CAD build for the part. Positions are in the model's coordinates, mm. A direction names the side the tool comes from. Coordinates: 2 decimals unless noted, no trailing zeros. Write each loop counter-clockwise with the first axis right and the second up, starting at its lowest first coordinate (ties: lowest second). Pieces come first, ordered by that corner, then holes. Notation, with made-up numbers: (18.25, 38) - (56.25, 38) arc R4 cw to (56.25, 44) - close; hole circle Ø6 at (17.5, -9). An arc over 180 degrees is marked (long way). Answer in a Markdown table with one row per item. Add a question column.
Q1. Band-saw the part on B-B (y = 9). List the corners of the cut face in (x, z), and give its area (3 significant figures).
Q2. Band-saw the part on C-C (z = 0). List the corners of the cut face in (x, y).
Q3. Drill centre lines: line 1 along X through (y, z) = (5.75, 0); line 2 along X through (y, z) = (2.75, 5.75); line 3 along Y through (x, z) = (16, 7). Where is each one in solid material? Low to high. Write a range as from..to.
Q4. Band-saw the part on A-A (x = 10). List the corners of the cut face in (y, z).
Q5. Two-plate mould, pull along Z, no slides. Class faces 5 (the cylindrical face through (4.5, 3, -7.5)), 6 (the flat face through (0, 1, 10)), 7 (the flat face through (-20, 1, 0)): +Z half, -Z half, draft (parallel to the pull), parting line (faces both ways), or undercut.
Q6. Pin check, flat tips, straight feed: pin 1 (6 mm diameter, centred on x = -11, y = 12, fed in from -Z); pin 2 (3.5 mm diameter, centred on x = 0, z = -8, fed in from +Y); pin 3 (4 mm diameter, centred on x = -11, z = -3.5, fed in from +Y). Stop position of each tip, or through.
Q7. 3-axis set-ups, long thin cutter, end or side, ignore diameter. For faces 1 (the cylindrical face through (-17.32, 7.92, -1.63)), 2 (the flat face through (0, 3, -9)), 3 (the flat face through (0, 4, -8)), 4 (the flat face through (20, 1, 0)): which of +Z, -Z, +X, -X, +Y, -Y reach the whole face in a straight line?
```python
from build123d import *

# Parameters (mm, degrees)
SKETCH1_W           = 40
SKETCH1_H           = 20
BOSS_EXTRUDE1_DEPTH = 2
SKETCH2_R           = 7.5
BOSS_EXTRUDE2_DEPTH = 12
SKETCH3_R           = 6.5
CUT_EXTRUDE1_DEPTH  = 12
SKETCH7_R           = 6.5
CUT_EXTRUDE2_DEPTH  = 12
BOSS_EXTRUDE3_DEPTH = 2


with BuildPart() as part:
    # Sketch1 → Boss-Extrude1 (new body)
    with BuildSketch(Plane(origin=(0, 0, 0), x_dir=(1, 0, 0), z_dir=(0, 1, 0))):
        Rectangle(SKETCH1_W, SKETCH1_H)
    extrude(amount=BOSS_EXTRUDE1_DEPTH)

    # Sketch2 → Boss-Extrude2 (add)
    with BuildSketch(Plane(origin=(0, 2, 0), x_dir=(1, 0, 0), z_dir=(0, 1, 0))):
        with Locations(Location((-10, 0, 0), (0, 0, 270))):
            Circle(SKETCH2_R)
        with Locations(Location((10, 0, 0), (0, 0, 270))):
            Circle(SKETCH2_R)
    extrude(amount=BOSS_EXTRUDE2_DEPTH)

    # Sketch3 → Cut-Extrude1 (cut)
    with BuildSketch(Plane(origin=(0, 14, 0), x_dir=(1, 0, 0), z_dir=(0, 1, 0))):
        with Locations(Location((-10, 0, 0), (0, 0, 270))):
            Circle(SKETCH3_R)
    extrude(amount=-CUT_EXTRUDE1_DEPTH, mode=Mode.SUBTRACT)

    # Sketch7 → Cut-Extrude2 (cut)
    with BuildSketch(Plane(origin=(0, 14, 0), x_dir=(1, 0, 0), z_dir=(0, 1, 0))):
        with Locations(Location((10, 0, 0), (0, 0, 270))):
            Circle(SKETCH7_R)
    extrude(amount=-CUT_EXTRUDE2_DEPTH, mode=Mode.SUBTRACT)

    # Sketch9 → Boss-Extrude3 (add)
    with BuildSketch(Plane(origin=(0, 2, 0), x_dir=(1, 0, 0), z_dir=(0, 1, 0))):
        with BuildLine():
            Line((-3, 9), (3, 9))
            ThreePointArc((3, 9), (4.5, 7.5), (3, 6))
            Line((3, 6), (-3, 6))
            ThreePointArc((-3, 6), (-4.5, 7.5), (-3, 9))
        make_face()
    extrude(amount=BOSS_EXTRUDE3_DEPTH)


solid = part.part
```
Checked values:
| question | item | result |
|---|---|---|
| 1 | outline | circle Ø15 at (-10, 0); circle Ø15 at (10, 0); hole circle Ø13 at (-10, 0); hole circle Ø13 at (10, 0) |
| 1 | area | 88.0 mm² |
| 2 | outline | (-20, 0) - (20, 0) - (20, 2) - (17.5, 2) - (17.5, 14) - (16.5, 14) - (16.5, 2) - (3.5, 2) - (3.5, 14) - (2.5, 14) - (2.5, 2) - (-2.5, 2) - (-2.5, 14) - (-3.5, 14) - (-3.5, 2) - (-16.5, 2) - (-16.5, 14) - (-17.5, 14) - (-17.5, 2) - (-20, 2) - close |
| 3 | line 1 | x = -17.5..-16.5, -3.5..-2.5, 2.5..3.5, 16.5..17.5 |
| 3 | line 2 | x = -14.82..-13.03, -6.97..-5.18, 5.18..6.97, 13.03..14.82 |
| 3 | line 3 | y = 0..2 |
| 4 | outline | (0, -10) - (2, -10) - (2, -7.5) - (14, -7.5) - (14, -6.5) - (2, -6.5) - (2, 6.5) - (14, 6.5) - (14, 7.5) - (2, 7.5) - (2, 10) - (0, 10) - close |
| 5 | face 5 | undercut |
| 5 | face 6 | +Z half |
| 5 | face 7 | draft |
| 6 | pin 1 | stops at z = -7.5 |
| 6 | pin 2 | stops at y = 4 |
| 6 | pin 3 | stops at y = 2 |
| 7 | face 1 | +Y |
| 7 | face 2 | -Z, +X, -X, +Y |
| 7 | face 3 | -Z, +Y |
| 7 | face 4 | +Z, -Z, +X, +Y, -Y |
